from build123d import *

# Parameters (mm, degrees)
F1_DEPTH = 2414
F2_W     = 92.1814972758
F2_H     = 150
F2_W_2   = 70
F2_W_3   = 4
F3_DEPTH = 141.501
F4_DEPTH = 139
F5_DEPTH = 139
F6_W     = 50
F6_H     = 2
F7_DEPTH = 25


with BuildPart() as f1:
    # F0 (on Top) → F1 (new body)
    with BuildSketch(Plane.XY):
        with BuildLine():
            Line((-55.2241730846, 112.5), (-59.2241730846, 112.5))
            Line((-59.2241730846, 112.5), (-59.2241730846, 4))
            ThreePointArc((-59.2241730846, 4), (-58.0526002093, 1.1715728753), (-55.2241730846, 0))
            Line((-55.2241730846, 0), (49.7758269154, 0))
            ThreePointArc((49.7758269154, 0), (52.6042540402, 1.1715728753), (53.7758269154, 4))
            Line((53.7758269154, 4), (53.7758269154, 141.5))
            Line((53.7758269154, 141.5), (48.7758269154, 141.5))
            Line((48.7758269154, 141.5), (48.7758269154, 8))
            ThreePointArc((48.7758269154, 8), (47.6042540402, 5.1715728753), (44.7758269154, 4))
            Line((44.7758269154, 4), (-51.2241730846, 4))
            ThreePointArc((-51.2241730846, 4), (-54.0526002093, 5.1715728753), (-55.2241730846, 8))
            Line((-55.2241730846, 8), (-55.2241730846, 112.5))
        make_face()
    extrude(amount=F1_DEPTH)

    # F2 (on face) → F3 (cut, through all)
    with BuildSketch(Plane.XZ):
        with Locations((99.8665755533, 2339)):
            Rectangle(F2_W, F2_H)
        with Locations((14.7758269154, 2339)):
            Rectangle(F2_W_2, F2_H)
        with Locations((51.7758269154, 2339)):
            Rectangle(F2_W_3, F2_H)
        with Locations((51.7758269154, 75)):
            Rectangle(F2_W_3, F2_H)
        with Locations((99.8665755533, 75)):
            Rectangle(F2_W, F2_H)
        with Locations((14.7758269154, 75)):
            Rectangle(F2_W_2, F2_H)
    extrude(amount=-F3_DEPTH, mode=Mode.SUBTRACT)

    # F4 (cut): a face of the model
    f4_faces = [f1.faces().sort_by_distance(p)[0] for p in [
        (-21.4148556619, 2, 2414),
    ]]
    extrude(f4_faces, amount=-F4_DEPTH, mode=Mode.SUBTRACT)

    # F5 (cut): a face of the model
    f5_faces = [f1.faces().sort_by_distance(p)[0] for p in [
        (-21.4148556619, 2, 0),
    ]]
    extrude(f5_faces, amount=-F5_DEPTH, mode=Mode.SUBTRACT)

    # F6 (on face) → F7 (cut)
    with BuildSketch(Plane.YZ.offset(-55.2241730846)):
        Polygon((50, 139), (112.5, 139), (112.5, 222), (50, 222), (50, 141), align=None)
        with Locations((25, 140)):
            Rectangle(F6_W, F6_H)
        Polygon((112.5, 2192), (112.5, 2275), (50, 2275), (50, 2273), (50, 2192), align=None)
        with Locations((25, 2274)):
            Rectangle(F6_W, F6_H)
    extrude(amount=-F7_DEPTH, mode=Mode.SUBTRACT)


solid = f1.part
The listing builds one solid part. Answer for the finished solid, in the listing's coordinates (mm). A direction names the side the tool comes from. Give positions to 0.01 mm unless a question says otherwise; leave off trailing zeros. Write each loop counter-clockwise with the first axis right and the second up, starting at its lowest first coordinate (ties: lowest second). Pieces come first, ordered by that corner, then holes. Notation, with made-up numbers: (-26.75, -3) -> (8.25, -3) arc R26 ccw to (8.25, 21) -> close; hole circle Ø5 at (63.5, 80). An arc over 180 degrees is marked (long way). One line per question, with ' | ' between items. Start each with the question number.
1. Find the intervals of material crossed by probe 1 along X at (y, z) = (66, 937.5); probe 2 along X at (y, z) = (113.5, 1215); probe 3 along Y at (x, z) = (-2, 1749.5), in increasing order.
2. Section B-B (z = 1164.5) is taken. Determine the outline of the cut face in (x, y).
3. Section C-C (x = 19.5) is taken. Determine the outline of the cut face in (y, z), plus the area to 3 significant figures.
4. Section A-A (y = 67.5) is taken. Determine the outline of the cut face in (x, z), plus the area to 4 significant figures.
5. For a pull along X with two mould halves and no side action, classify faces 1 (the flat face through (48.776, 76, 1192)), 2 (the flat face through (50, 49, 150)), 3 (the flat face through (53.776, 72, 1192)), 4 (the flat face through (-3, 4, 1192)) as pulls with the +X half, pulls with the -X half, needs draft (parallel to the pull), parting line crosses it, or undercut.
6. Given pin 1 Ø2 at (x, z) = (-58, 857) entering from +Y; pin 2 Ø1.5 at (x, z) = (35.5, 1034) entering from +Y; pin 3 Ø3 at (x, y) = (-57, 20.5) entering from -Z, each flat-ended and moving along its own axis, determine where each tip first touches the part or whether it passes through.
7. For faces 5 (the flat face through (49, 49, 2264)), 6 (the flat face through (-55.224, 60, 1192)), 7 (the flat face through (-59.224, 59, 1192)), determine the directions among +Z, -Z, +X, -X, +Y, -Y from which every point of the face is accessible in a straight line to the end or side of a thin tool.
Response values:
1) probe 1: -59.22 to -55.22, 48.78 to 53.78 | probe 2: 48.78 to 53.78 | probe 3: 0 to 4
2) outline: (-59.22, 4) arc R4 ccw to (-55.22, 0) -> (49.78, 0) arc R4 ccw to (53.78, 4) -> (53.78, 141.5) -> (48.78, 141.5) -> (48.78, 8) arc R4 cw to (44.78, 4) -> (-51.22, 4) arc R4 cw to (-55.22, 8) -> (-55.22, 112.5) -> (-59.22, 112.5) -> close
3) outline: (0, 150) -> (4, 150) -> (4, 2264) -> (0, 2264) -> close | area: 8,460 mm2
4) outline: (-59.22, 222) -> (-55.22, 222) -> (-55.22, 2192) -> (-59.22, 2192) -> close; (48.78, 150) -> (53.78, 150) -> (53.78, 2264) -> (48.78, 2264) -> close | area: 18,450 mm2
5) face 1: undercut | face 2: needs draft | face 3: pulls with the +X half | face 4: undercut
6) pin 1: y = 112.5 | pin 2: y = 4 | pin 3: z = 141
7) face 5: +Z, +X, +Y, -Y | face 6: +Z, -Z, +Y | face 7: +Z, -Z, -X, +Y, -Y
